Could you check a few things on this model? Use its own coordinates, in mm. Give positions to 0.01 mm unless a question says otherwise; leave off trailing zeros. Write each loop counter-clockwise with the first axis right and the second up, starting at its lowest first coordinate (ties: lowest second). Pieces come first, ordered by that corner, then holes. Notation, with made-up numbers: M 50.5,89 L 77.5,89 A13 cw 77.5,101 Z; hole C -26.5,74 d6. An arc over 180 degrees is marked long. Write each question's results on one line, items separated by ' | '. Start each with the question number.
from build123d import *

# Parameters (mm, degrees)
F0_W     = 76.2
F0_H     = 50.8
F0_R     = 3.175
F1_DEPTH = 31.75
F2_R     = 5.08
F4_DEPTH = 76.201


with BuildPart() as f1:
    # F0 (on Top) → F1 (new body)
    with BuildSketch(Plane.XY):
        Rectangle(F0_W, F0_H)
        with Locations((-28.575, -19.05)):
            Circle(F0_R, mode=Mode.SUBTRACT)
        with Locations((25.4, -16.933333)):
            Circle(F0_R, mode=Mode.SUBTRACT)
        with Locations((-25.4, 16.933333)):
            Circle(F0_R, mode=Mode.SUBTRACT)
        with Locations((28.575, 19.05)):
            Circle(F0_R, mode=Mode.SUBTRACT)
    extrude(amount=F1_DEPTH)

    # F2
    f2_edges = [f1.edges().sort_by_distance(p)[0] for p in [
        (-38.1, 25.4, 15.875),
        (-38.1, -25.4, 15.875),
        (38.1, 25.4, 15.875),
        (38.1, -25.4, 15.875),
    ]]
    fillet(f2_edges, radius=F2_R)

    # F3 (on face) → F4 (cut, through all)
    with BuildSketch(Plane(origin=(-38.1, 0, 0), x_dir=(0, -1, 0), z_dir=(-1, 0, 0))):
        with BuildLine():
            Line((-25.4, 0), (25.4, 0))
            ThreePointArc((25.4, 0), (0, 25.4), (-25.4, 0))
        make_face()
    extrude(amount=-F4_DEPTH, mode=Mode.SUBTRACT)


solid = f1.part
Q1. If we section it at B-B (z = 27): Please give me the cut outline in (x, y) (3 decimals).
Q2. I'm going to push flat-ended pins straight in: P1, Ø2, axis at x = 9, y = -12.5, coming from the -Z side; P2, Ø5, axis at x = 28.575, y = 19.05, coming from the -Z side; P3, Ø8.5, axis at x = 25.4, y = -16.93, coming from the -Z side; P4, Ø1, axis at x = 25, y = -8.5, coming from the -Z side. Where does each tip first touch, or does it pass through?
Q3. If we mould it in two halves opening along X, with no side actions, what happens to faces 1 (the face through (0, 25.4, 16)), 2 (the face through (38.1, 0, 27)), 3 (the face through (-25.81, 20.08, 25.32)), 4 (the face through (-35.98, -24.45, 19.63))? For each: pulls with the +X half, pulls with the -X half, needs draft (parallel to the pull), parting line crosses it, or undercut.
Q4. If we section it at A-A (y = -19.05): Please give me the cut outline in (x, z), plus the area to 3 significant figures.
Q5. If we section it at C-C (z = 5.5): Please give me the cut outline in (x, y).
Q6. If we section it at D-D (y = 0): Please give me the cut outline in (x, z), plus the area to 3 significant figures.
Q7. Please list where these lines run through material, in increasing order: line 1 (X direction, y = -19.5, z = 28.5); line 2 (X direction, y = -17, z = 26.5); line 3 (Y direction, x = -5, z = 23). Write a range as [from, to].
Determined:
1) outline: M -38.1,-20.32 A5.08 ccw -33.02,-25.4 L 33.02,-25.4 A5.08 ccw 38.1,-20.32 L 38.1,20.32 A5.08 ccw 33.02,25.4 L -33.02,25.4 A5.08 ccw -38.1,20.32 Z; hole C -28.575,-19.05 d6.35; hole C -25.4,16.933 d6.35; hole C 25.4,-16.933 d6.35; hole C 28.575,19.05 d6.35
2) P1: stops at z = 21.52 | P2: passes through | P3: stops at z = 14.02 | P4: stops at z = 23.75
3) face 1: needs draft | face 2: pulls with the +X half | face 3: undercut | face 4: pulls with the -X half
4) outline: M -38.1,16.8 L -31.75,16.8 L -31.75,31.75 L -38.1,31.75 Z; M -25.4,16.8 L 23.03,16.8 L 23.03,31.75 L -25.4,31.75 Z; M 27.77,16.8 L 38.1,16.8 L 38.1,31.75 L 27.77,31.75 Z | area: 973 mm²
5) outline: M -35.42,-24.8 A5.08 ccw -33.02,-25.4 L 33.02,-25.4 A5.08 ccw 35.42,-24.8 Z; M -35.42,24.8 L 35.42,24.8 A5.08 ccw 33.02,25.4 L -33.02,25.4 A5.08 ccw Z
6) outline: M -38.1,25.4 L 38.1,25.4 L 38.1,31.75 L -38.1,31.75 Z | area: 484 mm²
7) line 1: x = [-38.1, -31.72], [-25.43, 23.53], [27.27, 38.1] | line 2: x = [-38.1, -31], [-26.15, 22.23], [28.57, 38.1] | line 3: y = [-25.4, -10.78], [10.78, 25.4]
